Autodesk Inventor part; units mm, degrees
ref_plane "YZ Plane" through (0, 0, 0) normal (1, 0, 0) x (0, 1, 0)
ref_plane "XZ Plane" through (0, 0, 0) normal (0, 1, 0) x (-1, 0, 0)
ref_plane "XY Plane" through (0, 0, 0) normal (0, 0, 1) x (1, 0, 0)
sketch "Sketch1" plane through (0, 0, 0) normal (0, 1, 0) x (-1, 0, 0)
  line L0 (21.0733, 0) -> (10.5366, -18.25)
  line L1 (10.5366, -18.25) -> (-10.5366, -18.25)
  line L2 (-10.5366, -18.25) -> (-21.0733, 0)
  line L3 (-21.0733, 0) -> (-10.5366, 18.25)
  line L4 (-10.5366, 18.25) -> (10.5366, 18.25)
  line L5 (10.5366, 18.25) -> (21.0733, 0)
  line L6 (25.6921, 0) -> (12.846, -22.25)
  line L7 (12.846, -22.25) -> (-12.846, -22.25)
  line L8 (-12.846, -22.25) -> (-25.6921, 0)
  line L9 (-25.6921, 0) -> (-12.846, 22.25)
  line L10 (-12.846, 22.25) -> (12.846, 22.25)
  line L11 (12.846, 22.25) -> (25.6921, 0)
  line L12 (86.6025, 0) -> (43.3013, -75)
  line L13 (43.3013, -75) -> (-43.3013, -75)
  line L14 (-43.3013, -75) -> (-86.6025, 0)
  line L15 (-86.6025, 0) -> (-43.3013, 75)
  line L16 (-43.3013, 75) -> (43.3013, 75)
  line L17 (43.3013, 75) -> (86.6025, 0)
  point P0 (0, 0)
  point P1 (0, 0)
  dimension "d0" = 36.5
  dimension "d1" = 4
  dimension "d2" = 150
extrude "Extrusion1" add sketch "Sketch1" along normal blind 23 contours L6 L7 L8 L9 L10 L11
extrude "Extrusion2" add sketch "Sketch1" against normal blind 3 contours L0 L1 L2 L3 L4 L5 | L6 L7 L8 L9 L10 L11 | L12 L13 L14 L15 L16 L17
sketch "Sketch2" plane through (0, 0, 0) normal (0, 1, 0) x (1, 0, 0)
  circle A0 centre (0, 0) radius 9.85
  circle A1 centre (0, 0) radius 9
  dimension "d7" = 19.7
  dimension "d8" = 18
extrude "Extrusion3" [suppressed]
chamfer "Chamfer1" distance 0.5 angle 45 6 edges at (0, 23, 18.25) (-15.805, 23, 9.125) (-15.805, 23, -9.125) (0, 23, -18.25) (15.805, 23, -9.125) (15.805, 23, 9.125)
chamfer "Chamfer2" [suppressed]
properties part number "staender_tisch"
CAD build for the part. Positions are in the model's coordinates, mm. A direction names the side the tool comes from. Give positions to 0.01 mm unless a question says otherwise; leave off trailing zeros. Loops run counter-clockwise (first coordinate to the right, second up) from the corner with the lowest first, then second, coordinate; pieces in that order, holes last. Notation, with made-up numbers: (48.25, -28.75) - (73.25, -28.75) arc R25 cw to (73.25, -6.75) - close; hole circle Ø2 at (12, 23). An arc over 180 degrees is marked (long way). Put each result on its own line as item: value.
Q1. Slice it at B-B (x = 0). Give the cut face in (y, z).
Filled in:
outline: (-3, -75) - (0, -75) - (0, -22.25) - (23, -22.25) - (23, -18.75) - (22.5, -18.25) - (0, -18.25) - (0, 18.25) - (22.5, 18.25) - (23, 18.75) - (23, 22.25) - (0, 22.25) - (0, 75) - (-3, 75) - close
Q2. Probe line 1 along Z through (x, y) = (6.5, 4.75); line 2 along X through (y, z) = (6, -6); line 3 along Y through (x, z) = (71, 22). List the from-to ranges inside material, lowest first.
Filled in:
line 1: z = -22.25 to -18.25, 18.25 to 22.25
line 2: x = -22.23 to -17.61, 17.61 to 22.23
line 3: y = -3 to 0
Q3. Slice it at A-A (y = 18.5). Give the cut face in (x, z), plus the area to 3 significant figures.
Filled in:
outline: (-25.69, 0) - (-12.85, -22.25) - (12.85, -22.25) - (25.69, 0) - (12.85, 22.25) - (-12.85, 22.25) - close; hole (-21.07, 0) - (-10.54, -18.25) - (10.54, -18.25) - (21.07, 0) - (10.54, 18.25) - (-10.54, 18.25) - close
area: 561 mm²
Q4. Flat gauge pins, fed straight in: pin 1 (7 mm diameter, centred on x = -2.5, y = 9.5, fed in from +Z); pin 2 (11 mm diameter, centred on x = -3, z = -0.5, fed in from +Y); pin 3 (2 mm diameter, centred on x = 28.5, y = 7, fed in from +Z). Where does each tip first touch, or does it go through?
Filled in:
pin 1: stops at z = 22.25
pin 2: stops at y = 0
pin 3: passes through
Q5. Slice it at C-C (z = 9). Give the cut face in (x, y).
Filled in:
outline: (-81.41, -3) - (81.41, -3) - (81.41, 0) - (20.5, 0) - (20.5, 23) - (16.45, 23) - (15.88, 22.5) - (15.88, 0) - (-15.88, 0) - (-15.88, 22.5) - (-16.45, 23) - (-20.5, 23) - (-20.5, 0) - (-81.41, 0) - close
Q6. Mould opens along Z. For faces 5 (the face through (0, 11, -22.25)), 6 (the face through (19.36, 11.34, 10.97)), 7 (the face through (-15.943, 22.746, 9.379)), 8 (the face through (1, -3, 1)) say: pulls with the +Z half, pulls with the -Z half, needs draft (parallel to the pull), parting line crosses it, or undercut.
Filled in:
face 5: pulls with the -Z half
face 6: pulls with the +Z half
face 7: undercut
face 8: needs draft
Q7. Slice it at D-D (x = 53). Give the cut face in (y, z).
Filled in:
outline: (-3, -58.2) - (0, -58.2) - (0, 58.2) - (-3, 58.2) - close
Q8. Tool access for faces 1 (the face through (-19.36, 11.34, -10.97)), 2 (the face through (-19.18, 11.34, 11.28)), 3 (the face through (15.731, 11.092, -9.253)), 4 (the face through (0, 11, 22.25)): list every direction of +Z, -Z, +X, -X, +Y, -Y with a clear straight run to the whole face (end or side of a thin tool).
Filled in:
face 1: -Z, -X, +Y
face 2: +Z, -X, +Y
face 3: +Y
face 4: +Z, +X, -X, +Y
